```python
from build123d import *

# Parameters (mm, degrees)
F0_R     = 24.13
F1_DEPTH = 19.05
F2_R     = 25.4
F3_DEPTH = 38.1
F4_R     = 19.05
F5_DEPTH = 57.151


with BuildPart() as f1:
    # F0 (on Front) → F1 (new body)
    with BuildSketch(Plane.XZ):
        Circle(F0_R)
    extrude(amount=-F1_DEPTH)

    # F2 (on face) → F3 (join)
    with BuildSketch(Plane.XZ):
        Circle(F2_R)
    extrude(amount=F3_DEPTH)

    # F4 (on face) → F5 (cut, through all)
    with BuildSketch(Plane.XZ.offset(38.1)):
        Circle(F4_R)
    extrude(amount=-F5_DEPTH, mode=Mode.SUBTRACT)


solid = f1.part
```
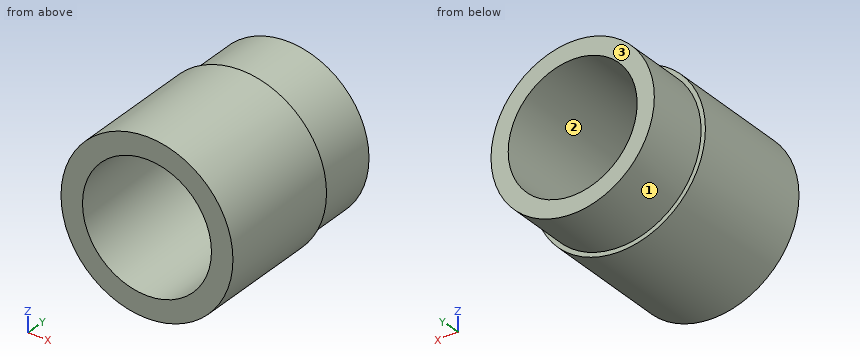
Geometry: final body of the model. Coordinates: model frame, mm. Face numbers are marked on the shaded views. Round coordinates to 2 decimals unless told otherwise and drop trailing zeros. Order: outer loops, then holes, each group sorted by start corner. A loop starts at its lowest first (then second) coordinate and runs counter-clockwise, first axis right, second up. Notation, with made-up numbers: (41, 27) -> (78, 27) arc R7 cw to (78, 33) -> close; hole circle Ø11 at (75.5, 45). An arc over 180 degrees is marked (long way). Use one line per item in the form item = value. Start each with the question number.
1. Cut plane D-D (z = 20.5). Return the cut outline in (x, y), then the cut area to 3 significant figures.
2. Cut plane B-B (z = 0). Return the cut outline in (x, y).
3. Line query: probe 1 along Z at (x, y) = (0, -26); probe 2 along X at (y, z) = (-6, 4.5); probe 3 along Z at (x, y) = (7, -33). Output: solid intervals per line, ascending.
4. Cut plane C-C (y = -26). Return the cut outline in (x, z).
5. Pin query (flat end, axial travel): pin 1 Ø1 at (y, z) = (-3, 10.5) entering from -X; pin 2 Ø1 at (x, y) = (11, 12.5) entering from +Z; pin 3 Ø3 at (x, y) = (-13, -23.5) entering from -Z; pin 4 Ø10 at (x, z) = (-10.5, -13.5) entering from -Y. Return the tip coordinate at first contact, or that it passes through.
6. Draft query along X for the marked faces 1, 2 and 3. Return one class per face: pulls with the +X half, pulls with the -X half, needs draft (parallel to the pull), parting line crosses it, or undercut.
7. Cut plane A-A (x = 0). Return the cut outline in (y, z), then the cut area to 3 significant figures.
Solution:
q1.outline = (-15, -38.1) -> (15, -38.1) -> (15, 0) -> (12.73, 0) -> (12.73, 19.05) -> (-12.73, 19.05) -> (-12.73, 0) -> (-15, 0) -> close
q1.area = 1,630 mm^2
q2.outline = (-25.4, -38.1) -> (-19.05, -38.1) -> (-19.05, 19.05) -> (-24.13, 19.05) -> (-24.13, 0) -> (-25.4, 0) -> close; (19.05, -38.1) -> (25.4, -38.1) -> (25.4, 0) -> (24.13, 0) -> (24.13, 19.05) -> (19.05, 19.05) -> close
q3.probe_1 = -25.4 to -19.05, 19.05 to 25.4
q3.probe_2 = -25 to -18.51, 18.51 to 25
q3.probe_3 = -24.42 to -17.72, 17.72 to 24.42
q4.outline = circle Ø50.8 at (0, 0); hole circle Ø38.1 at (0, 0)
q5.pin_1 = -23.35
q5.pin_2 = 21.73
q5.pin_3 = -22.65
q5.pin_4 = -38.1
q6.face_1 = parting line crosses it
q6.face_2 = undercut
q6.face_3 = needs draft
q7.outline = (-38.1, -25.4) -> (0, -25.4) -> (0, -24.13) -> (19.05, -24.13) -> (19.05, -19.05) -> (-38.1, -19.05) -> close; (-38.1, 19.05) -> (19.05, 19.05) -> (19.05, 24.13) -> (0, 24.13) -> (0, 25.4) -> (-38.1, 25.4) -> close
q7.area = 677 mm^2
